```python
from build123d import *

# Parameters (mm, degrees)
SKETCH1_W           = 67.31
SKETCH1_H           = 86.36
BOSS_EXTRUDE1_DEPTH = 19.05
SHELL1_T            = -3.81
FILLET3_R           = 10
CUT_EXTRUDE1_REACH  = 96.624
SKETCH2_R           = 2.0955


with BuildPart() as part:
    # Sketch1 → Boss-Extrude1 (new body)
    with BuildSketch(Plane.XY):
        Rectangle(SKETCH1_W, SKETCH1_H)
    extrude(amount=BOSS_EXTRUDE1_DEPTH)

    # Shell1
    shell1_openings = [part.faces().sort_by_distance(p)[0] for p in [
        (0, 0, 19.05),
    ]]
    offset(amount=SHELL1_T, openings=shell1_openings, kind=Kind.INTERSECTION)

    # Fillet3
    fillet3_edges = [part.edges().sort_by_distance(p)[0] for p in [
        (33.655, -43.18, 9.525),
        (-33.655, -43.18, 9.525),
        (-33.655, 43.18, 9.525),
        (33.655, 43.18, 9.525),
    ]]
    fillet(fillet3_edges, radius=FILLET3_R)

    # Sketch2 → Cut-Extrude1 (cut, up to next)
    with BuildSketch(Plane(origin=(0, 43.18, 0), x_dir=(1, 0, 0), z_dir=(0, 1, 0)), mode=Mode.PRIVATE) as cut_extrude1_sk1:
        with Locations(Location((0, -11.176, 0), (0, 0, 270))):
            Circle(SKETCH2_R)
    cut_extrude1_tool1 = extrude(cut_extrude1_sk1.sketch, amount=-CUT_EXTRUDE1_REACH, mode=Mode.PRIVATE) & part.part
    add(cut_extrude1_tool1.solids().sort_by_distance((0, 43.18, 11.176))[0], mode=Mode.SUBTRACT)


solid = part.part
```
Build history of the part. All positions in model axes, mm. A direction names the side the tool comes from. Give positions to 0.01 mm unless a question says otherwise; leave off trailing zeros. Loops run counter-clockwise (first coordinate to the right, second up) from the corner with the lowest first, then second, coordinate; pieces in that order, holes last. Notation, with made-up numbers: (-36.5, -18.75) -> (3.5, -18.75) arc R8 ccw to (3.5, -11.75) -> close; hole circle Ø5 at (35, 55.25). An arc over 180 degrees is marked (long way). One line per question, with ' | ' between items. Start each with the question number.
1) Pin check, flat tip, straight feed: pin 1 (3 mm diameter, centred on x = -12, y = 30.5, fed in from +Z). Stop position of the tip, or through.
2) Two-plate mould, pull along X, no slides. Class faces 4 (the flat face through (0, -43.18, 9)), 5 (the flat face through (-33.655, 0, 9)), 6 (the flat face through (0, 1, 3.81)): released by +X, released by -X, zero draft, split by the parting line, or undercut.
3) Probe L1, parallel to Y at x = 6, z = 10; L2, parallel to X at y = 20, z = 14.5 (3 decimals); L3, parallel to Z at x = -15, y = 27. List the from-to ranges inside material, lowest first.
4) Cut at A-A (x = 0). Give the cut face in (y, z).
5) Cut at B-B (y = -24). Give the cut face in (x, z) (3 decimals).
6) Cut at C-C (z = 5.25). Give the cut face in (x, y) (3 decimals), plus the area to 3 significant figures.
7) 3-axis set-ups, long thin cutter, end or side, ignore diameter. For faces 1 (the cylindrical face through (-0.803, 41.302, 13.112)), 2 (the flat face through (0, 39.37, 8)), 3 (the cylindrical face through (30.648, -40.328, 9.658)): which of +Z, -Z, +X, -X, +Y, -Y reach the whole face in a straight line?
8) Cut at D-D (x = -26). Give the cut face in (y, z), plus the area to 3 significant figures.
Return value:
1) pin 1: z = 3.81
2) face 4: zero draft | face 5: released by -X | face 6: undercut
3) L1: -43.18 to -39.37, 39.37 to 43.18 | L2: -33.655 to -29.845, 29.845 to 33.655 | L3: 0 to 3.81
4) outline: (-43.18, 0) -> (43.18, 0) -> (43.18, 9.08) -> (39.37, 9.08) -> (39.37, 3.81) -> (-39.37, 3.81) -> (-39.37, 19.05) -> (-43.18, 19.05) -> close; (39.37, 13.27) -> (43.18, 13.27) -> (43.18, 19.05) -> (39.37, 19.05) -> close
5) outline: (-33.655, 0) -> (33.655, 0) -> (33.655, 19.05) -> (29.845, 19.05) -> (29.845, 3.81) -> (-29.845, 3.81) -> (-29.845, 19.05) -> (-33.655, 19.05) -> close
6) outline: (-33.655, -33.18) arc R10 ccw to (-23.655, -43.18) -> (23.655, -43.18) arc R10 ccw to (33.655, -33.18) -> (33.655, 33.18) arc R10 ccw to (23.655, 43.18) -> (-23.655, 43.18) arc R10 ccw to (-33.655, 33.18) -> close; hole (-29.845, -39.37) -> (29.845, -39.37) -> (29.845, 39.37) -> (-29.845, 39.37) -> close | area: 1,030 mm^2
7) face 1: +Y | face 2: +Z | face 3: +Z, -Z, +X, -Y
8) outline: (-42.9, 0) -> (42.9, 0) -> (42.9, 19.05) -> (39.37, 19.05) -> (39.37, 3.81) -> (-39.37, 3.81) -> (-39.37, 19.05) -> (-42.9, 19.05) -> close | area: 435 mm^2
